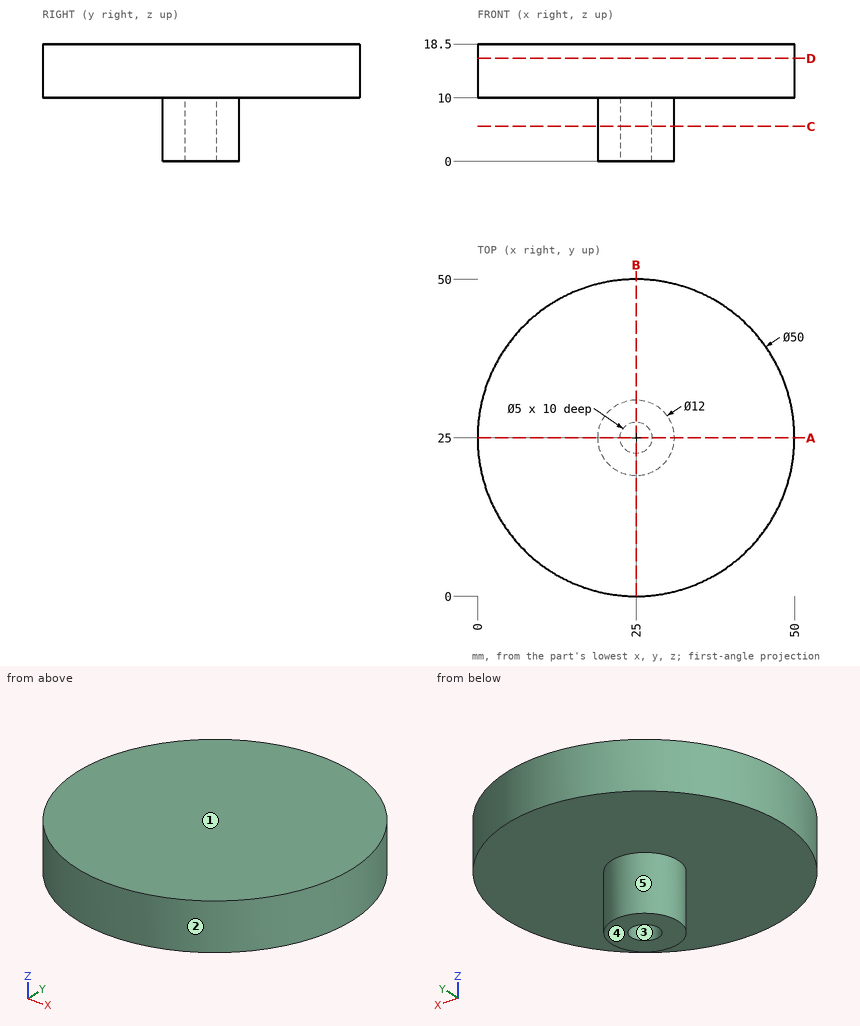
Study the drawing (mm; zero at the part's minimum x, y, z) and answer. A direction names the side the tool comes from. Round coordinates to 2 decimals unless told otherwise and drop trailing zeros. Loops run counter-clockwise (first coordinate to the right, second up) from the corner with the lowest first, then second, coordinate; pieces in that order, holes last. Notation, with made-up numbers: (-24.5, 4) -> (-19.5, 4) arc R36 cw to (-19.5, 43) -> close; hole circle Ø9 at (-17, -22.5). An arc over 180 degrees is marked (long way). Write each question's results on one line, items separated by ' | '. Start each with the question number.
1. Given pin 1 Ø6 at (y, z) = (38.5, 7.5) entering from -X; pin 2 Ø5 at (x, z) = (33, 7) entering from -Y; pin 3 Ø8 at (x, z) = (31.5, 8.5) entering from -Y, each flat-ended and moving along its own axis, determine where each tip first touches the part or whether it passes through.
2. Section D-D (z = 16.25) is taken. Determine the outline of the cut face in (x, y), plus the area to 3 significant figures.
3. For a pull along Y with two mould halves and no side action, classify the marked faces 1, 2 and 3 as +Y half, -Y half, draft (parallel to the pull), parting line (faces both ways), or undercut.
4. Section C-C (z = 5.5) is taken. Determine the outline of the cut face in (x, y), plus the area to 3 significant figures.
5. Section A-A (y = 25) is taken. Determine the outline of the cut face in (x, z), plus the area to 3 significant figures.
6. A tool of negligible diameter and unlimited length cuts with its end or side. For the marked faces 4 and 5, from which of +Z, -Z, +X, -X, +Y, -Y can it reach the whole face along a straight path? Write none if from no direction.
7. Find the intervals of material crossed by probe 1 along Y at (x, z) = (25, 5); probe 2 along Z at (x, y) = (33, 39); probe 3 along Y at (x, z) = (15.5, 14.75), in increasing order. Write a range as from..to.
Evaluation:
1) pin 1: stops at x = 2.98 | pin 2: stops at y = 22.6 | pin 3: stops at y = 0.16
2) outline: circle Ø50 at (25, 25) | area: 1,960 mm2
3) face 1: draft | face 2: parting line | face 3: undercut
4) outline: circle Ø12 at (25, 25); hole circle Ø5 at (25, 25) | area: 93.5 mm2
5) outline: (0, 10) -> (19, 10) -> (19, 0) -> (22.5, 0) -> (22.5, 10) -> (27.5, 10) -> (27.5, 0) -> (31, 0) -> (31, 10) -> (50, 10) -> (50, 18.5) -> (0, 18.5) -> close | area: 495 mm2
6) face 4: -Z, +X, -X, +Y, -Y | face 5: -Z
7) probe 1: y = 19..22.5, 27.5..31 | probe 2: z = 10..18.5 | probe 3: y = 1.88..48.12
